Part model, mm, in its own coordinate system. A direction names the side the tool comes from. Give positions to 0.01 mm unless a question says otherwise; leave off trailing zeros. Write each loop counter-clockwise with the first axis right and the second up, starting at its lowest first coordinate (ties: lowest second). Pieces come first, ordered by that corner, then holes. Notation, with made-up numbers: (-12.5, 55) - (16.5, 55) arc R17 ccw to (16.5, 79) - close; hole circle Ø11 at (12, -0.75). An arc over 180 degrees is marked (long way). Answer as a JSON object with one key per item and string values. Group by question number.
```python
from build123d import *

# Parameters (mm, degrees)
F1_DEPTH      = 25.4
F2_W          = 38.9676727355
F2_H          = 83.2322090864
F3_DEPTH      = 50.038
F6_START      = -0.254
F5_R          = 7.8901435138
F6_DEPTH      = 83.058
F8_DEPTH      = 47.1165622497
F8_DEPTH_BACK = 8.1488895142


with BuildPart() as f1:
    # F0 (on Top) → F1 (new body)
    with BuildSketch(Plane.XY):
        with BuildLine():
            Line((-27.6095401496, 71.7521590341), (-27.6095401496, -72.8592127562))
            Line((-27.6095401496, -72.8592127562), (-27.1735749765, -72.8592127562))
            ThreePointArc((-27.1735749765, -72.8592127562), (0, -100.0327877326), (27.1735749765, -72.8592127562))
            Line((27.1735749765, -72.8592127562), (27.6095401496, -72.8592127562))
            Line((27.6095401496, -72.8592127562), (27.6095401496, 71.7521590341))
            ThreePointArc((27.6095401496, 71.7521590341), (0, 100.4909386381), (-27.6095401496, 71.7521590341))
        make_face()
        with BuildLine():
            ThreePointArc((-12.7623392826, -72.8592127562), (0, -60.0968734736), (12.7623392826, -72.8592127562))
            ThreePointArc((12.7623392826, -72.8592127562), (0, -85.6215520387), (-12.7623392826, -72.8592127562))
        make_face(mode=Mode.SUBTRACT)
        with BuildLine():
            ThreePointArc((14.8305593579, 72.8592127562), (0, 58.0286533983), (-14.8305593579, 72.8592127562))
            ThreePointArc((-14.8305593579, 72.8592127562), (0, 87.689772114), (14.8305593579, 72.8592127562))
        make_face(mode=Mode.SUBTRACT)
    extrude(amount=F1_DEPTH)

    # F2 (on face) → F3 (join)
    with BuildSketch(Plane.XY.offset(25.4)):
        Rectangle(F2_W, F2_H)
    extrude(amount=F3_DEPTH)

    # F5 (on face) → F6 (join)
    with BuildSketch(Plane.XZ.offset(41.6161045432).offset(F6_START)):
        with BuildLine():
            ThreePointArc((19.4838363677, 74.4076669397), (21.5273694016, 79.5792249141), (22.2230663556, 85.0962027907))
            ThreePointArc((22.2230663556, 85.0962027907), (-5.5169778767, 106.6235721923), (-19.4838363677, 74.4076669397))
            Line((-19.4838363677, 74.4076669397), (-19.4838363677, 75.438))
            Line((-19.4838363677, 75.438), (19.4838363677, 75.438))
            Line((19.4838363677, 75.438), (19.4838363677, 74.4076669397))
        make_face()
        with Locations((0, 85.0962027907)):
            Circle(F5_R, mode=Mode.SUBTRACT)
    extrude(amount=-F6_DEPTH)

    # F7 (on face) → F8 (cut, two sides)
    with BuildSketch(Plane.YZ.offset(19.4838363677)) as f8_sk:
        with BuildLine():
            Line((24.7208084911, 53.0094616115), (24.7208084911, 74.4076669397))
            Line((24.7208084911, 74.4076669397), (-24.6291831136, 74.4076669397))
            Line((-24.6291831136, 74.4076669397), (-24.6291831136, 53.0094616115))
            ThreePointArc((-24.6291831136, 53.0094616115), (-17.2473636439, 36.4565333824), (0, 30.8870505542))
            ThreePointArc((0, 30.8870505542), (17.3054188168, 36.4224226696), (24.7208084911, 53.0094616115))
        make_face()
        Polygon((24.7208084911, 74.4076669397), (24.7208084911, 108.5037675067), (-24.6291831136, 108.1680555029), (-24.6291831136, 74.4076669397), align=None)
    extrude(amount=-F8_DEPTH, mode=Mode.SUBTRACT)
    extrude(f8_sk.sketch, amount=F8_DEPTH_BACK, mode=Mode.SUBTRACT)


solid = f1.part
```
1) Band-saw the part on A-A (z = 21). List the corners of the cut face in (x, y).
2) Band-saw the part on C-C (x = 0). State how many separate pieces and enclosed holes the cut face has, plus the area to 3 significant figures.
3) Probe line 1 (Z direction, x = 0.5, y = 26.5); line 2 (Y direction, x = -13, z = 66.5); line 3 (Y direction, x = -2, z = 102.5). List the from-to ranges inside material, lowest first.
4) Mould opens along X. For faces 4 (the cylindrical face through (3.641, 33.09, 78.096)), 5 (the flat face through (27.61, -2, 13)), 6 (the flat face through (0, 41.616, 50)) say: pulls with the +X half, pulls with the -X half, needs draft (parallel to the pull), parting line crosses it, or undercut.
5) Drop flat-ended pins along their axis: P1, Ø3, axis at y = 3, z = 30.5, coming from the +X side; P2, Ø2, axis at y = -70.5, z = 23.5, coming from the -X side; P3, Ø7.5, axis at y = -34, z = 7.5, coming from the +X side. Give the stop position or say it passes through.
6) Band-saw the part on B-B (y = 35). List the corners of the cut face in (x, z).
7) Which spindle directions (+Z, -Z, +X, -X, +Y, -Y) get a long thin tool onto all of the face, cutting with end or side? Do faces 1 (the flat face through (19.484, -1, 28)), 2 (the flat face through (0, -41.616, 50)), 3 (the flat face through (0, -24.629, 75)). Say none if no direction does.
8) Band-saw the part on D-D (z = 62). List the corners of the cut face in (x, y), plus the area to 3 significant figures.
Verdict:
{
 "1": {"outline": "(-27.61, -72.86) - (-27.17, -72.86) arc R27.17 ccw to (27.17, -72.86) - (27.61, -72.86) - (27.61, 71.75) arc R27.63 ccw (long way) to (-27.61, 71.75) - close; hole circle Ø29.66 at (0, 72.86); hole circle Ø25.52 at (0, -72.86)"},
 "2": {"separate pieces": "5", "enclosed holes": "0", "area": "6,410 mm2"},
 "3": {"line 1": "0 to 77.22, 92.97 to 107.31", "line 2": "-41.62 to -24.63, 24.72 to 41.62", "line 3": "-41.36 to -24.63, 24.72 to 41.7"},
 "4": {"face 4": "undercut", "face 5": "pulls with the +X half", "face 6": "needs draft"},
 "5": {"P1": "x = 19.48", "P2": "x = -27.61", "P3": "x = 27.61"},
 "6": {"outline": "(-27.61, 0) - (27.61, 0) - (27.61, 25.4) - (19.48, 25.4) - (19.48, 74.41) arc R22.22 ccw (long way) to (-19.48, 74.41) - (-19.48, 25.4) - (-27.61, 25.4) - close; hole circle Ø15.78 at (0, 85.1)"},
 "7": {"face 1": "+X, +Y, -Y", "face 2": "+Z, +X, -X, -Y", "face 3": "+Z, +X, -X"},
 "8": {"outline": "(-19.48, -41.62) - (19.48, -41.62) - (19.48, -24.63) - (-19.48, -24.63) - close; (-19.48, 24.72) - (19.48, 24.72) - (19.48, 41.62) - (-19.48, 41.62) - close", "area": "1,320 mm2"}
}
